```python
from build123d import *

# Parameters (mm, degrees)
IZIM1_R                     = 6
Y_KSEKLIK_EKSTR_ZYON1_DEPTH = 50
IZIM2_R                     = 5
Y_KSEKLIK_EKSTR_ZYON2_DEPTH = 16
IZIM3_R                     = 5
Y_KSEKLIK_EKSTR_ZYON3_DEPTH = 16


with BuildPart() as part:
    # Çizim1 → Yükseklik-Ekstrüzyon1 (new body)
    with BuildSketch(Plane(origin=(0, 0, 0), x_dir=(0, 0, -1), z_dir=(1, 0, 0))):
        Circle(IZIM1_R)
    extrude(amount=Y_KSEKLIK_EKSTR_ZYON1_DEPTH)

    # Çizim2 → Yükseklik-Ekstrüzyon2 (add)
    with BuildSketch(Plane.ZY):
        Circle(IZIM2_R)
    extrude(amount=Y_KSEKLIK_EKSTR_ZYON2_DEPTH)

    # Çizim3 → Yükseklik-Ekstrüzyon3 (add)
    with BuildSketch(Plane(origin=(50, 0, 0), x_dir=(0, 0, -1), z_dir=(1, 0, 0))):
        Circle(IZIM3_R)
    extrude(amount=Y_KSEKLIK_EKSTR_ZYON3_DEPTH)


solid = part.part
```
Source: CAD feature listing. Evaluate the final solid. Frame: model axes, mm. A direction names the side the tool comes from. Coordinates: 2 decimals unless noted, no trailing zeros. Order: outer loops, then holes, each group sorted by start corner. A loop starts at its lowest first (then second) coordinate and runs counter-clockwise, first axis right, second up. Notation, with made-up numbers: M -23.75,28.5 L -8.75,28.5 A26 cw -8.75,48.5 Z; hole C -40,-14.5 d7. An arc over 180 degrees is marked long. Write each question's results on one line, items separated by ' | '. Start each with the question number.
1) Section query B-B (z = -4.25). Return the cut outline in (x, y), plus the area to 3 significant figures.
2) Section query D-D (x = 44). Return the cut outline in (y, z).
3) Access query for faces 1 (the face through (-7.89, -4.88, -1.08)), 2 (the face through (25, 0, 6)), 3 (the face through (50, 4, 4)). Directions: +Z, -Z, +X, -X, +Y, -Y. A direction counts if a zero-diameter tool reaches every point of the face in a straight line with its end or side. Return the directions, or none.
4) Section query C-C (x = -3). Return the cut outline in (y, z), plus the area to 3 significant figures.
5) Line query: line 1 (X direction, y = 0.75, z = 5.25); line 2 (Y direction, x = 3, z = -0.75). Output: solid intervals per line, ascending. Write a range as from..to.
6) Section query A-A (y = 0). Return the cut outline in (x, z), plus the area to 3 significant figures.
7) Contact query for flat-ended pins moving along their axis: pin 1 Ø1 at (x, z) = (51, 1.5) entering from +Y; pin 2 Ø2 at (x, z) = (9, -4.5) entering from -Y; pin 3 Ø3 at (x, y) = (46.5, 4.5) entering from -Z. Output: stop coordinate, or through.
Answers:
1) outline: M -16,-2.63 L 0,-2.63 L 0,-4.24 L 50,-4.24 L 50,-2.63 L 66,-2.63 L 66,2.63 L 50,2.63 L 50,4.24 L 0,4.24 L 0,2.63 L -16,2.63 Z | area: 592 mm^2
2) outline: C 0,0 d12
3) face 1: -X | face 2: +X, -X | face 3: +X
4) outline: C 0,0 d10 | area: 78.5 mm^2
5) line 1: x = 0..50 | line 2: y = -5.95..5.95
6) outline: M -16,-5 L 0,-5 L 0,-6 L 50,-6 L 50,-5 L 66,-5 L 66,5 L 50,5 L 50,6 L 0,6 L 0,5 L -16,5 Z | area: 920 mm^2
7) pin 1: stops at y = 4.9 | pin 2: stops at y = -4.87 | pin 3: stops at z = -5.2
